Model file for the job. Use its own axes, mm. Round coordinates to 2 decimals unless told otherwise and drop trailing zeros. Order: outer loops, then holes, each group sorted by start corner. A loop starts at its lowest first (then second) coordinate and runs counter-clockwise, first axis right, second up. Notation, with made-up numbers: (-35.75, 26.25) - (13.25, 26.25) arc R14 ccw to (13.25, 31.25) - close; hole circle Ø2 at (13.5, -19.75). An arc over 180 degrees is marked (long way). Answer as CSV lines item,"result". Start each with the question number.
1. Band-saw the part on B-B on z = 4.25. State how many separate pieces and enclosed holes the cut face has, then the cut area to 3 significant figures.
2. Pull direction Y, two halves, no side cores. Call faces 1 (the face through (3.119, 0.693, 3.949)), 2 (the face through (4.46, 0.46, 3.95)), 3 (the face through (0, 0, 0)), 4 (the face through (5.669, -2.035, 4.056)): released by +Y, released by -Y, zero draft, split by the parting line, or undercut.
3. Band-saw the part on A-A on x = 0.93. List the corners of the cut face in (y, z), then the cut area to 3 significant figures.
4. Pin check, flat tip, straight feed: pin 1 Ø1 at (y, z) = (1.5, 7) entering from +X. Stop position of the tip, or through.
5. Wall check: line 1 along Y through (x, z) = (-0.88, 2.5); line 2 along Y through (x, z) = (4.55, 4); line 3 along X through (y, z) = (-1.4, 2.5). Give the ranges that are in metal, low to high. Write a range as [from, to].
6. Band-saw the part on D-D on y = -1.9. List the corners of the cut face in (x, z).
```python
from build123d import *

# Parameters (mm, degrees)
SKETCH_W     = 11.94
SKETCH_H     = 4.64
SKETCH_R     = 0.34
SKETCH_R_2   = 0.45
SKETCH_R_3   = 0.44
SKETCH_R_4   = 0.43
SKETCH_R_5   = 0.42
SKETCH_R_6   = 0.41
SKETCH_R_7   = 0.4
SKETCH_R_8   = 0.35
SKETCH_R_9   = 0.36
SKETCH_R_10  = 0.37
SKETCH_R_11  = 0.38
SKETCH_R_12  = 0.39
PAD_DEPTH    = 8
CHAMFER_SIZE = 0.34
FILLET_R     = 1


with BuildPart() as part:
    # Sketch → Pad (new body)
    with BuildSketch(Plane.XY):
        Rectangle(SKETCH_W, SKETCH_H)
        with Locations((-4.5, -0.96)):
            Circle(SKETCH_R, mode=Mode.SUBTRACT)
        with Locations((-4.5, 0.85)):
            Circle(SKETCH_R_2, mode=Mode.SUBTRACT)
        with Locations((-2.69, 0.85)):
            Circle(SKETCH_R_3, mode=Mode.SUBTRACT)
        with Locations((-0.88, 0.85)):
            Circle(SKETCH_R_4, mode=Mode.SUBTRACT)
        with Locations((0.93, 0.85)):
            Circle(SKETCH_R_5, mode=Mode.SUBTRACT)
        with Locations((2.74, 0.85)):
            Circle(SKETCH_R_6, mode=Mode.SUBTRACT)
        with Locations((4.55, 0.85)):
            Circle(SKETCH_R_7, mode=Mode.SUBTRACT)
        with Locations((-2.69, -0.96)):
            Circle(SKETCH_R_8, mode=Mode.SUBTRACT)
        with Locations((-0.88, -0.96)):
            Circle(SKETCH_R_9, mode=Mode.SUBTRACT)
        with Locations((0.93, -0.96)):
            Circle(SKETCH_R_10, mode=Mode.SUBTRACT)
        with Locations((2.74, -0.96)):
            Circle(SKETCH_R_11, mode=Mode.SUBTRACT)
        with Locations((4.55, -0.96)):
            Circle(SKETCH_R_12, mode=Mode.SUBTRACT)
    extrude(amount=PAD_DEPTH)

    # Chamfer
    chamfer_edges = [part.edges().sort_by_distance(p)[0] for p in [
        (-4.16, -0.96, 4),
        (-4.84, -0.96, 0),
        (-4.84, -0.96, 8),
        (-4.05, 0.85, 4),
        (-4.95, 0.85, 0),
        (-4.95, 0.85, 8),
        (-2.25, 0.85, 4),
        (-3.13, 0.85, 0),
        (-3.13, 0.85, 8),
        (-2.34, -0.96, 4),
        (-3.04, -0.96, 0),
        (-3.04, -0.96, 8),
        (-0.45, 0.85, 4),
        (-1.31, 0.85, 0),
        (-1.31, 0.85, 8),
        (-0.52, -0.96, 4),
        (-1.24, -0.96, 0),
        (-1.24, -0.96, 8),
        (1.35, 0.85, 4),
        (0.51, 0.85, 0),
        (0.51, 0.85, 8),
        (1.3, -0.96, 4),
        (0.56, -0.96, 0),
        (0.56, -0.96, 8),
        (3.15, 0.85, 4),
        (2.33, 0.85, 0),
        (2.33, 0.85, 8),
        (3.12, -0.96, 4),
        (2.36, -0.96, 0),
        (2.36, -0.96, 8),
        (4.95, 0.85, 4),
        (4.15, 0.85, 0),
        (4.15, 0.85, 8),
        (4.94, -0.96, 4),
        (4.16, -0.96, 0),
        (4.16, -0.96, 8),
    ]]
    chamfer(chamfer_edges, length=CHAMFER_SIZE)

    # Fillet
    fillet_edges = [part.edges().sort_by_distance(p)[0] for p in [
        (5.97, -2.32, 4),
        (5.97, 2.32, 4),
        (-5.97, -2.32, 4),
        (-5.97, 2.32, 4),
    ]]
    fillet(fillet_edges, radius=FILLET_R)


solid = part.part
```
Reply:
1,separate pieces,"1"
1,enclosed holes,"12"
1,area,"48.6 mm2"
2,face 1,"undercut"
2,face 2,"undercut"
2,face 3,"zero draft"
2,face 4,"released by -Y"
3,outline,"(-2.32, 0) - (-1.67, 0) - (-1.33, 0.34) - (-1.33, 7.66) - (-1.67, 8) - (-2.32, 8) - close; (-0.59, 0.34) - (-0.25, 0) - (0.09, 0) - (0.43, 0.34) - (0.43, 7.66) - (0.09, 8) - (-0.25, 8) - (-0.59, 7.66) - close; (1.27, 0.34) - (1.61, 0) - (2.32, 0) - (2.32, 8) - (1.61, 8) - (1.27, 7.66) - close"
3,area,"24.0 mm2"
4,pin 1,"stops at x = 5.97"
5,line 1,"y = [-2.32, -1.32], [-0.6, 0.42], [1.28, 2.32]"
5,line 2,"y = [-2.32, -1.35], [-0.57, 0.45], [1.25, 2.32]"
5,line 3,"x = [-5.97, 5.97]"
6,outline,"(-5.78, 0) - (5.78, 0) - (5.78, 8) - (-5.78, 8) - close"
